Design review of the part shown in the three views and the two pictorial views. Dimensions are in mm from the part's minimum x, y and z. A direction names the side the tool comes from. Round coordinates to 2 decimals unless told otherwise and drop trailing zeros. Loops run counter-clockwise (first coordinate to the right, second up) from the corner with the lowest first, then second, coordinate; pieces in that order, holes last. Notation, with made-up numbers: M -38.75,42 L -32.75,42 A15 ccw -32.75,62 Z; hole C 77,74 d6. An arc over 180 degrees is marked long. One line per question, with ' | ' between items.
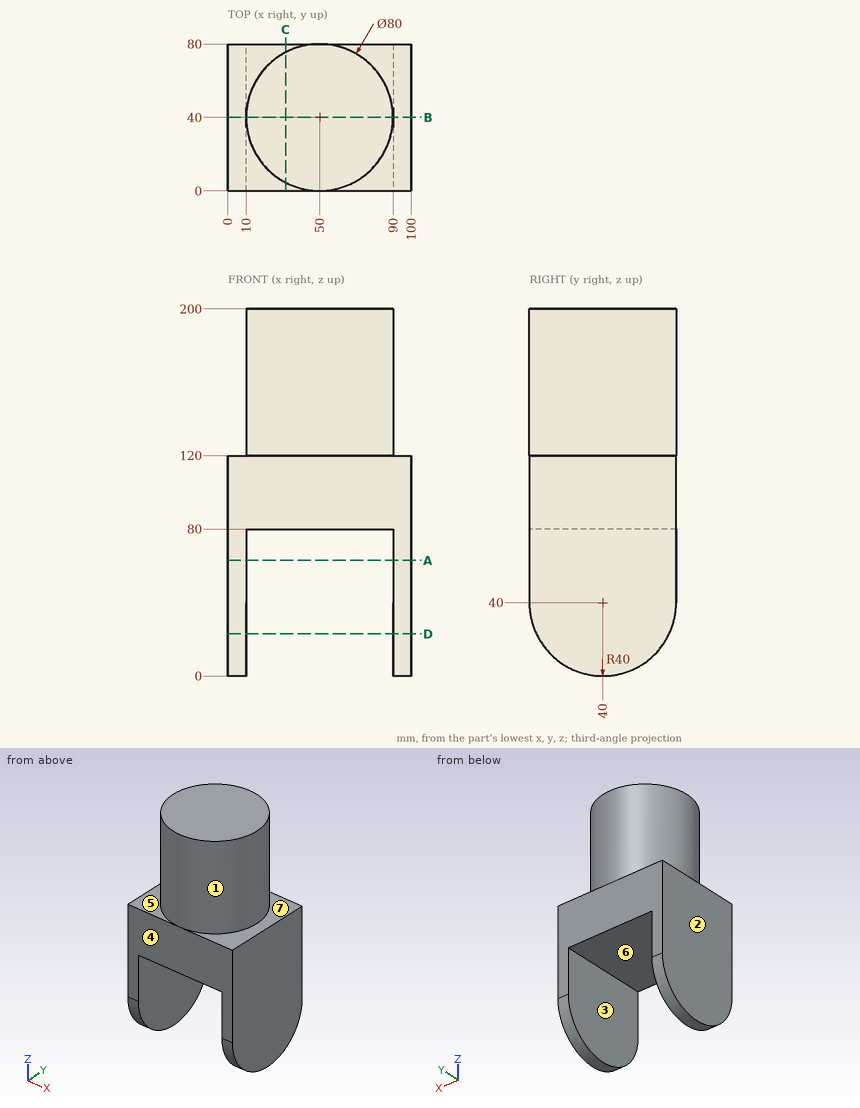
1) Add section B-B on y = 40. State the section outline as (x, z) points.
Output values:
outline: M 0,0 L 10,0 L 10,80 L 90,80 L 90,0 L 100,0 L 100,120 L 90,120 L 90,200 L 10,200 L 10,120 L 0,120 Z
2) For line 1 (X direction, y = 16, z = 74); line 2 (Z direction, x = 11.5, y = 49); line 3 (Z direction, x = 33, y = 76.5), list the stretches that pass through material, from the lowest coordinate up.
Output values:
line 1: x = 0 to 10, 90 to 100 | line 2: z = 80 to 200 | line 3: z = 80 to 120
3) Add section A-A on z = 63. State the section outline as (x, y) points, then the cut area to 3 significant figures.
Output values:
outline: M 0,0 L 10,0 L 10,80 L 0,80 Z; M 90,0 L 100,0 L 100,80 L 90,80 Z | area: 1,600 mm²
4) Add section D-D on z = 23. State the section outline as (x, y) points.
Output values:
outline: M 0,3.79 L 10,3.79 L 10,76.21 L 0,76.21 Z; M 90,3.79 L 100,3.79 L 100,76.21 L 90,76.21 Z
5) Add section C-C on x = 31.5. State the section outline as (y, z) points.
Output values:
outline: M 0,80 L 80,80 L 80,120 L 75.46,120 L 75.46,200 L 4.54,200 L 4.54,120 L 0,120 Z
6) Machinability: for the marked faces 5, 6 and 7, which of the approach directions +Z, -Z, +X, -X, +Y, -Y give a long, thin tool a straight path to every point of the face, cutting with its end or side? Answer none if there is none.
Output values:
face 5: +Z, -X | face 6: -Z, +Y, -Y | face 7: +Z, +X
7) Insertion check: P1, Ø1, axis at y = 55.5, z = 160, coming from the +X side; P2, Ø1.5, axis at x = 54, z = 132.5, coming from the -Y side; P3, Ø5, axis at y = 31.5, z = 177.5, coming from the +X side. Each pin has a flat end and moves straight along its axis. Give the tip position at first contact, or say it passes through.
Output values:
P1: stops at x = 87.08 | P2: stops at y = 0.13 | P3: stops at x = 89.55
8) Mouldability with a two-part tool opening along X and no side actions: class the marked faces 1, 2, 3 and 4 as +X half, -X half, draft (parallel to the pull), parting line (faces both ways), or undercut.
Output values:
face 1: parting line | face 2: -X half | face 3: undercut | face 4: draft
